Input: part model. Units: mm. Frame: model coordinates. A direction names the side the tool comes from. Coordinates: 2 decimals unless noted, no trailing zeros. Order: outer loops, then holes, each group sorted by start corner. A loop starts at its lowest first (then second) coordinate and runs counter-clockwise, first axis right, second up. Notation, with made-up numbers: (-5, -16) -> (29, -16) arc R19 ccw to (29, 0) -> close; hole circle Ø7 at (8, 62.25). An arc over 180 degrees is marked (long way). Answer as CSV lines item,"result".
from build123d import *

# Parameters (mm, degrees)
ESBO_O1_R                = 7.8
ESBO_O1_R_2              = 3.05
RESSALTO_EXTRUS_O1_DEPTH = 9.1
ESBO_O2_R                = 9.3
ESBO_O2_R_2              = 7.8
RESSALTO_EXTRUS_O2_DEPTH = 1
RESSALTO_EXTRUS_O3_START = -1
ESBO_O3_R                = 9.3
ESBO_O3_R_2              = 7.8
RESSALTO_EXTRUS_O3_DEPTH = 1


with BuildPart() as part:
    # Esboço1 → Ressalto-extrusão1 (new body)
    with BuildSketch(Plane.XY):
        Circle(ESBO_O1_R)
        Circle(ESBO_O1_R_2, mode=Mode.SUBTRACT)
    extrude(amount=RESSALTO_EXTRUS_O1_DEPTH)

    # Esboço2 → Ressalto-extrusão2 (add)
    with BuildSketch(Plane(origin=(0, 0, 0), x_dir=(-1, 0, 0), z_dir=(0, 0, -1))):
        Circle(ESBO_O2_R)
        Circle(ESBO_O2_R_2, mode=Mode.SUBTRACT)
    extrude(amount=-RESSALTO_EXTRUS_O2_DEPTH)

    # Esboço3 → Ressalto-extrusão3 (add)
    with BuildSketch(Plane.XY.offset(9.1).offset(RESSALTO_EXTRUS_O3_START)):
        with Locations(Location((0, 0, 0), (0, 0, 180))):
            Circle(ESBO_O3_R)
        with Locations(Location((0, 0, 0), (0, 0, 180))):
            Circle(ESBO_O3_R_2, mode=Mode.SUBTRACT)
    extrude(amount=RESSALTO_EXTRUS_O3_DEPTH)


solid = part.part
1. Cut plane D-D (y = 7.25). Return the cut outline in (x, z).
Findings:
outline,"(-5.82, 0) -> (5.82, 0) -> (5.82, 1) -> (2.88, 1) -> (2.88, 8.1) -> (5.82, 8.1) -> (5.82, 9.1) -> (-5.82, 9.1) -> (-5.82, 8.1) -> (-2.88, 8.1) -> (-2.88, 1) -> (-5.82, 1) -> close"
2. Reachability of faces 1 (the face through (-5.75, 5.27, 4.5)), 2 (the face through (-4, 0, 0)) from +Z, -Z, +X, -X, +Y, -Y: full face, straight path, thin tool, end or side. Return the list, or none.
Findings:
face 1,"none"
face 2,"-Z, +X, -X, +Y, -Y"
3. Cut plane A-A (x = 0). Return the cut outline in (y, z).
Findings:
outline,"(-9.3, 0) -> (-3.05, 0) -> (-3.05, 9.1) -> (-9.3, 9.1) -> (-9.3, 8.1) -> (-7.8, 8.1) -> (-7.8, 1) -> (-9.3, 1) -> close; (3.05, 0) -> (9.3, 0) -> (9.3, 1) -> (7.8, 1) -> (7.8, 8.1) -> (9.3, 8.1) -> (9.3, 9.1) -> (3.05, 9.1) -> close"
4. Contact query for flat-ended pins moving along their axis: pin 1 (4 mm diameter, centred on x = -3.5, z = 1.5, fed in from -Y); pin 2 (2 mm diameter, centred on y = 2.5, z = 5.5, fed in from -X); pin 3 (1.5 mm diameter, centred on x = -1, z = 3.5, fed in from +Y). Output: stop coordinate, or through.
Findings:
pin 1,"stops at y = -9.17"
pin 2,"stops at x = -7.65"
pin 3,"stops at y = 7.8"
5. Mould query, pull axis Z, two halves, no side actions, for faces 3 (the face through (-5, -7.84, 8.59)), 4 (the face through (-4, 0, 9.1)), 5 (the face through (-2, -8, 1)). Classes: released by +Z, released by -Z, zero draft, split by the parting line, or undercut.
Findings:
face 3,"zero draft"
face 4,"released by +Z"
face 5,"undercut"
6. Cut plane C-C (z = 6). Return the cut outline in (x, y).
Findings:
outline,"circle Ø15.6 at (0, 0); hole circle Ø6.1 at (0, 0)"
7. Ray query, line 1 along Y through (x, z) = (0, 4); line 2 along Z through (x, y) = (-6.5, -4.75); line 3 along X through (y, z) = (-1.5, 4.5). Return the intervals inside material, ascending.
Findings:
line 1,"y = -7.8 to -3.05, 3.05 to 7.8"
line 2,"z = 0 to 1, 8.1 to 9.1"
line 3,"x = -7.65 to -2.66, 2.66 to 7.65"
